Work out the finished part from the listing and answer in its coordinate system (mm). A direction names the side the tool comes from. Coordinates: 2 decimals unless noted, no trailing zeros. Order: outer loops, then holes, each group sorted by start corner. A loop starts at its lowest first (then second) coordinate and runs counter-clockwise, first axis right, second up.
```python
from build123d import *

# Parameters (mm, degrees)
BOSS_EXTRUDE1_DEPTH = 2
SKETCH1_3_W         = 30
SKETCH1_3_H         = 18
BOSS_EXTRUDE2_DEPTH = 20
CUT_EXTRUDE1_DEPTH  = 54.104524665


with BuildPart() as part:
    # Sketch1 → Boss-Extrude1 (new body)
    with BuildSketch(Plane(origin=(0, 0, 0), x_dir=(1, 0, 0), z_dir=(0, 1, 0))):
        Polygon((-14.414477612, 14.528955224), (-32.014477612, 14.528955224), (-32.014477612, -5.471044776), (32.585522388, -5.471044776), (32.585522388, 14.528955224), (15.585522388, 14.528955224), (15.585522388, -3.471044776), (-14.414477612, -3.471044776), align=None)
    extrude(amount=BOSS_EXTRUDE1_DEPTH)

    # Sketch1<3> → Boss-Extrude2 (add)
    with BuildSketch(Plane(origin=(0, 0, 0), x_dir=(1, 0, 0), z_dir=(0, 1, 0))):
        with Locations((0.585522388, 5.528955224)):
            Rectangle(SKETCH1_3_W, SKETCH1_3_H)
    extrude(amount=BOSS_EXTRUDE2_DEPTH)

    # Sketch2 → Cut-Extrude1 (cut, through all)
    with BuildSketch(Plane.ZY.offset(14.414477612)):
        with BuildLine():
            Line((-14.528955224, 20), (-14.528955224, 11))
            ThreePointArc((-14.528955224, 11), (-11.892916255, 17.363961031), (-5.528955224, 20))
            Line((-5.528955224, 20), (-14.528955224, 20))
        make_face()
        with BuildLine():
            ThreePointArc((-5.528955224, 20), (0.835005807, 17.363961031), (3.471044776, 11))
            Line((3.471044776, 11), (3.471044776, 20))
            Line((3.471044776, 20), (-5.528955224, 20))
        make_face()
    extrude(amount=-CUT_EXTRUDE1_DEPTH, mode=Mode.SUBTRACT)


solid = part.part
```
1. Consider probe 1 along Y at (x, z) = (-29, -7); probe 2 along X at (y, z) = (8, 1); probe 3 along Z at (x, y) = (2, 10). Determine where each line is inside the solid, lowest interval first.
2. For faces 1 (the flat face through (0, 6, 3.471)), 2 (the flat face through (15.586, 11, -5)), 3 (the flat face through (-14.414, 11, -5)), 4 (the flat face through (-32.014, 1, -5)), 5 (the flat face through (0, 4, -14.529)), determine the directions among +Z, -Z, +X, -X, +Y, -Y from which every point of the face is accessible in a straight line to the end or side of a thin tool.
3. The part is cut by section A-A (x = -3). Determine the outline of the cut face in (y, z), plus the area to 3 significant figures.
4. The part is cut by section B-B (z = -4.5). Determine the outline of the cut face in (x, y).
5. The part is cut by section C-C (y = 18.5). Determine the outline of the cut face in (x, z), plus the area to 3 significant figures.
6. The part is cut by section D-D (z = 2.5). Determine the outline of the cut face in (x, y).
7. Flat-ended cylindrical pins translate along their axes: pin 1 (10 mm diameter, centred on y = 11.5, z = -5.5, fed in from +X); pin 2 (6 mm diameter, centred on x = -9.5, z = -4.5, fed in from +Y); pin 3 (7 mm diameter, centred on x = 2, y = 8.5, fed in from +Z); pin 4 (8 mm diameter, centred on y = 8, z = -9, fed in from -X). Find the tip coordinate at first contact, or state that the pin passes through.
Worked out:
1. probe 1: y = 0 to 2
1. probe 2: x = -14.41 to 15.59
1. probe 3: z = -14.53 to 3.47
2. face 1: +Z, +X, -X, +Y
2. face 2: +Z, -Z, +X, +Y
2. face 3: +Z, -Z, -X, +Y
2. face 4: +Z, -Z, -X, +Y, -Y
2. face 5: -Z, +X, -X, +Y, -Y
3. outline: (0, -14.53) - (11, -14.53) arc R9 ccw to (11, 3.47) - (2, 3.47) - (2, 5.47) - (0, 5.47) - close
3. area: 329 mm2
4. outline: (-32.01, 0) - (32.59, 0) - (32.59, 2) - (15.59, 2) - (15.59, 19.94) - (-14.41, 19.94) - (-14.41, 2) - (-32.01, 2) - close
5. outline: (-14.41, -10.5) - (15.59, -10.5) - (15.59, -0.55) - (-14.41, -0.55) - close
5. area: 298 mm2
6. outline: (-32.01, 0) - (32.59, 0) - (32.59, 2) - (15.59, 2) - (15.59, 15.07) - (-14.41, 15.07) - (-14.41, 2) - (-32.01, 2) - close
7. pin 1: stops at x = 15.59
7. pin 2: stops at y = 20
7. pin 3: stops at z = 3.47
7. pin 4: stops at x = -14.41
